```python
from build123d import *

# Parameters (mm, degrees)
SKETCH1_W            = 184
SKETCH1_H            = 258
BOSS_EXTRUDE1_DEPTH  = 3
M5_CLEARANCE_HOLE1_D = 5.5
CUT_EXTRUDE1_DEPTH   = 10
M4_CLEARANCE_HOLE1_D = 4.5
LPATTERN1_COUNT      = 2
LPATTERN1_PITCH      = 60
LPATTERN2_COUNT      = 2
LPATTERN2_PITCH      = 170
SKETCH7_W            = 3
SKETCH7_H            = 100
CUT_EXTRUDE2_DEPTH   = 10


with BuildPart() as part:
    # Sketch1 → Boss-Extrude1 (new body)
    with BuildSketch(Plane.XY):
        with Locations((92, 129)):
            Rectangle(SKETCH1_W, SKETCH1_H)
    extrude(amount=BOSS_EXTRUDE1_DEPTH)

    # M5 Clearance Hole1 (through all)
    with Locations(Plane(origin=(0, 0, 0), x_dir=(-1, 0, 0), z_dir=(0, 0, -1))):
        with Locations((-175, 75), (-5, 134.225), (-5, 79.6125), (-175, 245), (-5, 25)):
            Hole(M5_CLEARANCE_HOLE1_D / 2)

    # Sketch4 → Cut-Extrude1 (cut)
    with BuildSketch(Plane(origin=(0, 0, 0), x_dir=(-1, 0, 0), z_dir=(0, 0, -1))):
        with BuildLine():
            Line((-61.767766953, 239.767766953), (-71.767766953, 229.767766953))
            ThreePointArc((-71.767766953, 229.767766953), (-71.767766953, 226.232233047), (-68.232233047, 226.232233047))
            Line((-68.232233047, 226.232233047), (-58.232233047, 236.232233047))
            ThreePointArc((-58.232233047, 236.232233047), (-58.232233047, 239.767766953), (-61.767766953, 239.767766953))
        make_face()
        with BuildLine():
            Line((-51.767766953, 239.767766953), (-71.767766953, 219.767766953))
            ThreePointArc((-71.767766953, 219.767766953), (-71.767766953, 216.232233047), (-68.232233047, 216.232233047))
            Line((-68.232233047, 216.232233047), (-48.232233047, 236.232233047))
            ThreePointArc((-48.232233047, 236.232233047), (-48.232233047, 239.767766953), (-51.767766953, 239.767766953))
        make_face()
        with BuildLine():
            Line((-41.767766953, 239.767766953), (-71.767766953, 209.767766953))
            ThreePointArc((-71.767766953, 209.767766953), (-71.767766953, 206.232233047), (-68.232233047, 206.232233047))
            Line((-68.232233047, 206.232233047), (-38.232233047, 236.232233047))
            ThreePointArc((-38.232233047, 236.232233047), (-38.232233047, 239.767766953), (-41.767766953, 239.767766953))
        make_face()
        with BuildLine():
            Line((-31.767766953, 239.767766953), (-71.767766953, 199.767766953))
            ThreePointArc((-71.767766953, 199.767766953), (-71.767766953, 196.232233047), (-68.232233047, 196.232233047))
            Line((-68.232233047, 196.232233047), (-28.232233047, 236.232233047))
            ThreePointArc((-28.232233047, 236.232233047), (-28.232233047, 239.767766953), (-31.767766953, 239.767766953))
        make_face()
        with BuildLine():
            ThreePointArc((-22.828427125, 231.636038969), (-22.828427125, 235.171572875), (-26.363961031, 235.171572875))
            Line((-26.363961031, 235.171572875), (-67.171572875, 194.363961031))
            ThreePointArc((-67.171572875, 194.363961031), (-67.171572875, 190.828427125), (-63.636038969, 190.828427125))
            Line((-63.636038969, 190.828427125), (-22.828427125, 231.636038969))
        make_face()
        with BuildLine():
            Line((-21.767766953, 229.767766953), (-61.767766953, 189.767766953))
            ThreePointArc((-61.767766953, 189.767766953), (-61.767766953, 186.232233047), (-58.232233047, 186.232233047))
            Line((-58.232233047, 186.232233047), (-18.232233047, 226.232233047))
            ThreePointArc((-18.232233047, 226.232233047), (-18.232233047, 229.767766953), (-21.767766953, 229.767766953))
        make_face()
        with BuildLine():
            Line((-48.232233047, 186.232233047), (-18.232233047, 216.232233047))
            ThreePointArc((-18.232233047, 216.232233047), (-18.232233047, 219.767766953), (-21.767766953, 219.767766953))
            Line((-21.767766953, 219.767766953), (-51.767766953, 189.767766953))
            ThreePointArc((-51.767766953, 189.767766953), (-51.767766953, 186.232233047), (-48.232233047, 186.232233047))
        make_face()
        with BuildLine():
            Line((-21.767766953, 209.767766953), (-41.767766953, 189.767766953))
            ThreePointArc((-41.767766953, 189.767766953), (-41.767766953, 186.232233047), (-38.232233047, 186.232233047))
            Line((-38.232233047, 186.232233047), (-18.232233047, 206.232233047))
            ThreePointArc((-18.232233047, 206.232233047), (-18.232233047, 209.767766953), (-21.767766953, 209.767766953))
        make_face()
        with BuildLine():
            Line((-21.767766953, 199.767766953), (-31.767766953, 189.767766953))
            ThreePointArc((-31.767766953, 189.767766953), (-31.767766953, 186.232233047), (-28.232233047, 186.232233047))
            Line((-28.232233047, 186.232233047), (-18.232233047, 196.232233047))
            ThreePointArc((-18.232233047, 196.232233047), (-18.232233047, 199.767766953), (-21.767766953, 199.767766953))
        make_face()
    cut_extrude1 = extrude(amount=-CUT_EXTRUDE1_DEPTH, mode=Mode.SUBTRACT)

    # M4 Clearance Hole1 (through all)
    with Locations(Plane(origin=(0, 0, 0), x_dir=(-1, 0, 0), z_dir=(0, 0, -1))):
        with Locations((-20, 188), (-70, 188), (-70, 238), (-20, 238)):
            m4_clearance_hole1 = Hole(M4_CLEARANCE_HOLE1_D / 2)

    # LPattern1: Cut-Extrude1, M4 Clearance Hole1 ×2
    with Locations(*[(0, -i * LPATTERN1_PITCH, 0) for i in range(1, LPATTERN1_COUNT)]):
        add(cut_extrude1, mode=Mode.SUBTRACT)
        add(m4_clearance_hole1, mode=Mode.SUBTRACT)

    # LPattern2: Cut-Extrude1, M4 Clearance Hole1 ×2
    with Locations(*[(0, -i * LPATTERN2_PITCH, 0) for i in range(1, LPATTERN2_COUNT)]):
        add(cut_extrude1, mode=Mode.SUBTRACT)
        add(m4_clearance_hole1, mode=Mode.SUBTRACT)

    # Sketch7 → Cut-Extrude2 (cut)
    with BuildSketch(Plane(origin=(0, 0, 0), x_dir=(-1, 0, 0), z_dir=(0, 0, -1))):
        with Locations((-182.5, 50)):
            Rectangle(SKETCH7_W, SKETCH7_H)
    extrude(amount=-CUT_EXTRUDE2_DEPTH, mode=Mode.SUBTRACT)


solid = part.part
```
Geometry: final body of the model. Coordinates: model frame, mm. Round coordinates to 2 decimals unless told otherwise and drop trailing zeros. Write each loop counter-clockwise with the first axis right and the second up, starting at its lowest first coordinate (ties: lowest second). Pieces come first, ordered by that corner, then holes. Notation, with made-up numbers: M -23.75,49.25 L -14.75,49.25 A26 ccw -14.75,73.25 Z; hole C 57,0.25 d3. An arc over 180 degrees is marked long. Answer in a Markdown table with one row per item. Add a question column.
(1) Contact query for flat-ended pins moving along their axis: pin 1 (8 mm diameter, centred on x = 96.5, y = 180, fed in from -Z); pin 2 (1.5 mm diameter, centred on x = 182.5, z = 1, fed in from -Y); pin 3 (0.9 mm diameter, centred on y = 28.5, z = 1, fed in from +X); pin 4 (2.5 mm diameter, centred on x = 20, y = 178, fed in from -Z). Output: stop coordinate, or through.
(2) Draft query along X for faces 1 (the face through (56.558, 224.978, 1.479)), 2 (the face through (33.442, 201.022, 1.479)). Return one class per face: pulls with the +X half, pulls with the -X half, needs draft (parallel to the pull), parting line crosses it, or undercut.
(3) Ray query, L1, parallel to Y at x = 175, z = 1.5; L2, parallel to X at y = 225, z = 0.2; L3, parallel to X at y = 87, z = 1.85. Return the intervals inside material, ascending.
(4) Cut plane A-A, the plane y = 245. Return the cut outline in (x, z), then the cut area to 4 significant figures.
(5) Cut plane B-B, the plane z = 2.3. Give the number of separate pieces and of enclosed holes in the cut face, then the cut area to 3 significant figures.
Established:
| question | item | result |
|---|---|---|
| 1 | pin 1 | z = 0 |
| 1 | pin 2 | y = 100 |
| 1 | pin 3 | x = 181 |
| 1 | pin 4 | through |
| 2 | face 1 | undercut |
| 2 | face 2 | undercut |
| 3 | L1 | 0 to 72.25, 77.75 to 242.25, 247.75 to 258 |
| 3 | L2 | 0 to 19.46, 26.54 to 29.46, 36.54 to 39.46, 46.54 to 49.46, 56.54 to 59.46, 66.54 to 184 |
| 3 | L3 | 0 to 181 |
| 4 | outline | M 0,0 L 172.25,0 L 172.25,3 L 0,3 Z; M 177.75,0 L 184,0 L 184,3 L 177.75,3 Z |
| 4 | area | 535.5 mm² |
| 5 | separate pieces | 1 |
| 5 | enclosed holes | 44 |
| 5 | area | 41,200 mm² |
